Autodesk Inventor part; units mm, degrees
ref_plane "YZ Plane" through (0, 0, 0) normal (1, 0, 0) x (0, 1, 0)
ref_plane "XZ Plane" through (0, 0, 0) normal (0, 1, 0) x (-1, 0, 0)
ref_plane "XY Plane" through (0, 0, 0) normal (0, 0, 1) x (1, 0, 0)
sketch "Sketch1" plane through (0, 0, 0) normal (0, 1, 0) x (-1, 0, 0)
  line L0 (0, 0) -> (12.7, 0)
  line L1 (12.7, 0) -> (12.7, -101.6)
  line L2 (12.7, -101.6) -> (0, -101.6)
  line L3 (0, -101.6) -> (0, 0)
  dimension "d1" = 12.7
  dimension "d2" = 101.6
extrude "Extrusion1" add sketch "Sketch1" along normal blind 107.95
sketch "Sketch2" plane through (0, 0, 0) normal (0, -1, 0) x (1, 0, 0)
  line L0 (0, 0) -> (0, -101.6)
  line L1 (0, -101.6) -> (0, -87.63)
  line L2 (0, 0) -> (0, -13.97)
  line L3 (0, -13.97) -> (-6.35, -13.97)
  line L4 (-6.35, -13.97) -> (-6.35, -25.4)
  line L5 (-6.35, -25.4) -> (0, -25.4)
  line L6 (0, -25.4) -> (0, -13.97)
  line L7 (0, -87.63) -> (-6.35, -87.63)
  line L8 (-6.35, -87.63) -> (-6.35, -76.2)
  line L9 (-6.35, -76.2) -> (0, -76.2)
  line L10 (0, -76.2) -> (0, -87.63)
  dimension "d6" = 13.97
  dimension "d9" = 13.97
  dimension "d10" = 6.35
  dimension "d11" = 11.43
  dimension "d12" = 6.35
  dimension "d13" = 11.43
extrude "Extrusion2" add sketch "Sketch2" along normal blind 25.4
sketch "Sketch3" plane through (0, 0, -101.6) normal (1, 0, 0) x (0, 0, -1)
  line L0 (-101.6, 0) -> (-101.6, 107.95)
  line L1 (-101.6, 107.95) -> (-76.2, 107.95)
  line L2 (0, 107.95) -> (-101.6, 107.95)
  line L3 (-76.2, 107.95) -> (-76.2, 101.6)
  line L4 (-76.2, 101.6) -> (-88.9, 101.6)
  line L5 (-88.9, 101.6) -> (-88.9, 104.775)
  line L6 (-88.9, 104.775) -> (-76.2, 104.775)
  line L7 (-76.2, 104.775) -> (-76.2, 101.6)
  line L8 (0, 107.95) -> (-25.4, 107.95)
  line L9 (-25.4, 107.95) -> (-25.4, 101.6)
  line L10 (-25.4, 101.6) -> (-12.7, 101.6)
  line L11 (-12.7, 101.6) -> (-12.7, 104.775)
  line L12 (-12.7, 104.775) -> (-25.4, 104.775)
  line L13 (-25.4, 104.775) -> (-25.4, 101.6)
  dimension "d17" = 25.4
  dimension "d18" = 6.35
  dimension "d19" = 12.7
  dimension "d20" = 3.175
  dimension "d21" = 25.4
  dimension "d22" = 6.35
  dimension "d23" = 12.7
  dimension "d24" = 3.175
extrude "Extrusion3" cut sketch "Sketch3" against normal blind 12.7
sketch "Sketch4" plane through (0, 0, -101.6) normal (1, 0, 0) x (0, 0, -1)
  line L0 (-75.6651, 101.8589) -> (-75.6651, 95.5089)
  line L1 (-75.6651, 95.5089) -> (-62.9651, 95.5089)
  line L2 (-62.9651, 95.5089) -> (-37.5651, 95.5089)
  line L3 (-37.5651, 95.5089) -> (-37.5651, 101.8589)
  line L4 (-37.5651, 101.8589) -> (-62.9651, 101.8589)
  line L5 (-62.9651, 101.8589) -> (-62.9651, 95.5089)
  point P0 (-101.6, 0)
  dimension "d29" = 6.35
  dimension "d30" = 12.7
  dimension "d31" = 25.4
  dimension "d32" = 6.35
extrude "Extrusion4" cut sketch "Sketch4" against normal blind 12.7
properties part number "back" material "LCP Plastic"
Input: part model. Units: mm. Frame: model coordinates. A direction names the side the tool comes from. Give positions to 0.01 mm unless a question says otherwise; leave off trailing zeros. Order: outer loops, then holes, each group sorted by start corner. A loop starts at its lowest first (then second) coordinate and runs counter-clockwise, first axis right, second up.
1. Set-up query: faces 1 (the face through (-6, 99, -38.635)), 2 (the face through (-3, -13, -76.2)), 3 (the face through (-3, -13, -87.63)). Return all of +Z, -Z, +X, -X, +Y, -Y with unobstructed straight access to the full face (end or side cutting, diameter ignored); none if empty.
Computed:
face 1: +X, -X
face 2: +X, -X, -Y
face 3: -Z, +X, -X, -Y
2. Cut plane D-D (z = -47). Return loops of the section in (x, y).
Computed:
outline: (-12.7, 0) - (0, 0) - (0, 95.51) - (-12.7, 95.51) - close; (-12.7, 101.86) - (0, 101.86) - (0, 107.95) - (-12.7, 107.95) - close
3. Cut plane C-C (y = -16). Return loops of the section in (x, z).
Computed:
outline: (-6.35, -87.63) - (0, -87.63) - (0, -76.2) - (-6.35, -76.2) - close; (-6.35, -25.4) - (0, -25.4) - (0, -13.97) - (-6.35, -13.97) - close
4. Line query: probe 1 along Y at (x, z) = (-2.5, -45); probe 2 along Y at (x, z) = (-6, -78) (3 decimals); probe 3 along Z at (x, y) = (-6, -17.5). Output: solid intervals per line, ascending.
Computed:
probe 1: y = 0 to 95.51, 101.86 to 107.95
probe 2: y = -25.4 to 101.6, 104.775 to 107.95
probe 3: z = -87.63 to -76.2, -25.4 to -13.97
5. Draft query along Z for faces 4 (the face through (-3, -25.4, -82)), 5 (the face through (-3, -13, -25.4)), 6 (the face through (-6, 53, 0)). Return one class per face: released by +Z, released by -Z, zero draft, split by the parting line, or undercut.
Computed:
face 4: zero draft
face 5: undercut
face 6: released by +Z
6. Cut plane B-B (x = -2.75). Return loops of the section in (y, z) (3 decimals).
Computed:
outline: (-25.4, -87.63) - (0, -87.63) - (0, -101.6) - (107.95, -101.6) - (107.95, 0) - (0, 0) - (0, -13.97) - (-25.4, -13.97) - (-25.4, -25.4) - (0, -25.4) - (0, -76.2) - (-25.4, -76.2) - close; hole (95.509, -64.035) - (101.859, -64.035) - (101.859, -38.635) - (95.509, -38.635) - close; hole (101.6, -88.9) - (104.775, -88.9) - (104.775, -76.2) - (101.6, -76.2) - close; hole (101.6, -25.4) - (104.775, -25.4) - (104.775, -12.7) - (101.6, -12.7) - close
7. Pin query (flat end, axial travel): pin 1 Ø6 at (y, z) = (57, -54.5) entering from +X; pin 2 Ø7 at (x, y) = (-2, -7.5) entering from -Z; pin 3 Ø9 at (y, z) = (-8.5, -84) entering from -X; pin 4 Ø5 at (x, z) = (-11, -61.5) entering from -Y. Return the tip coordinate at first contact, or that it passes through.
Computed:
pin 1: stops at x = 0
pin 2: stops at z = -87.63
pin 3: stops at x = -6.35
pin 4: stops at y = 0
8. Cut plane A-A (z = -21). Return loops of the section in (x, y) (3 decimals), and give its area (3 significant figures).
Computed:
outline: (-12.7, 0) - (-6.35, 0) - (-6.35, -25.4) - (0, -25.4) - (0, 101.6) - (-12.7, 101.6) - close; (-12.7, 104.775) - (0, 104.775) - (0, 107.95) - (-12.7, 107.95) - close
area: 1,490 mm2
